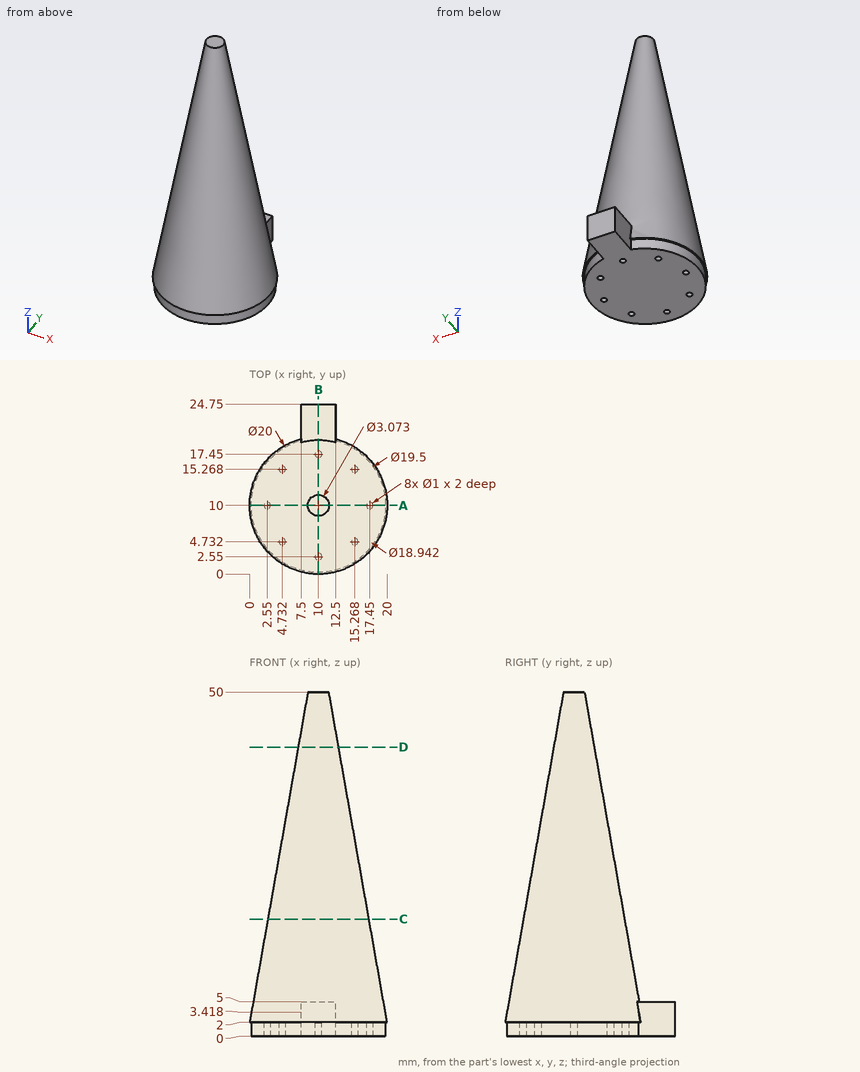
For this review, use the dimensioned drawing (mm, ordinates from the lowest corner) and the shaded views. Coordinates: 2 decimals unless noted, no trailing zeros. Write each loop counter-clockwise with the first axis right and the second up, starting at its lowest first coordinate (ties: lowest second). Pieces come first, ordered by that corner, then holes. Notation, with made-up numbers: (65.5, -8.75) - (118.5, -8.75) arc R21 ccw to (118.5, -3.75) - close; hole circle Ø7 at (72.5, -5.75). An arc over 180 degrees is marked (long way). One line per item, written item: value.
1) To check wall thickness, follow probe 1 along Y at (x, z) = (10, 0.5); probe 2 along X at (y, z) = (7.5, 23); probe 3 along Z at (x, y) = (12, 22). State the ranges of each line that lie inside material, in increasing order.
Answer sheet:
probe 1: y = 0.25 to 2.05, 3.05 to 16.95, 17.95 to 24.75
probe 2: x = 4.22 to 15.78
probe 3: z = 0 to 5
2) Insertion check: pin 1 (0.5 mm diameter, centred on x = 5, y = 15.5, fed in from -Z); pin 2 (1.5 mm diameter, centred on y = 22, z = 2.5, fed in from -X); pin 3 (5 mm diameter, centred on y = 6.5, z = 7.5, fed in from +X); pin 4 (8 mm diameter, centred on y = 13, z = 24, fed in from -X). Each pin has a flat end and moves straight along its axis. Give the tip position at first contact, or say it passes through.
Answer sheet:
pin 1: stops at z = 0
pin 2: stops at x = 7.5
pin 3: stops at x = 19.18
pin 4: stops at x = 3.34
3) Add section B-B (x = 10). State the section outline as (y, z) points, plus the area to 3 significant figures.
Answer sheet:
outline: (0, 2) - (0.25, 2) - (0.25, 0) - (2.05, 0) - (2.05, 2) - (3.05, 2) - (3.05, 0) - (16.95, 0) - (16.95, 2) - (17.95, 2) - (17.95, 0) - (24.75, 0) - (24.75, 5) - (19.47, 5) - (11.54, 50) - (8.46, 50) - close
area: 614 mm2
4) Add section C-C (z = 17). State the section outline as (x, y) points (1 decimal).
Answer sheet:
outline: circle Ø14.7 at (10, 10)
5) Add section A-A (y = 10). State the section outline as (x, z) points.
Answer sheet:
outline: (0, 2) - (0.25, 2) - (0.25, 0) - (2.05, 0) - (2.05, 2) - (3.05, 2) - (3.05, 0) - (16.95, 0) - (16.95, 2) - (17.95, 2) - (17.95, 0) - (19.75, 0) - (19.75, 2) - (20, 2) - (11.54, 50) - (8.46, 50) - close
6) Add section D-D (z = 42). State the section outline as (x, y) points, plus the area to 3 significant figures.
Answer sheet:
outline: circle Ø5.89 at (10, 10)
area: 27.3 mm2
